from build123d import *

# Parameters (mm, degrees)
SKETCH1_W           = 15.24
SKETCH1_H           = 20.066
SKETCH1_W_2         = 5.588
SKETCH1_H_2         = 9.906
BOSS_EXTRUDE1_DEPTH = 3.175
CUT_EXTRUDE1_REACH  = 14.993
SKETCH2_R           = 1.3


with BuildPart() as part:
    # Sketch1 → Boss-Extrude1 (new body)
    with BuildSketch(Plane.XY):
        Rectangle(SKETCH1_W, SKETCH1_H)
        Rectangle(SKETCH1_W_2, SKETCH1_H_2, mode=Mode.SUBTRACT)
    extrude(amount=BOSS_EXTRUDE1_DEPTH)

    # Sketch2 → Cut-Extrude1 (cut, up to next)
    with BuildSketch(Plane.XY.offset(3.175), mode=Mode.PRIVATE) as cut_extrude1_sk1:
        with Locations((-5.207, 7.112)):
            Circle(SKETCH2_R)
    cut_extrude1_tool1 = extrude(cut_extrude1_sk1.sketch, amount=-CUT_EXTRUDE1_REACH, mode=Mode.PRIVATE) & part.part
    # Sketch2 → Cut-Extrude1 (cut, up to next)
    with BuildSketch(Plane.XY.offset(3.175), mode=Mode.PRIVATE) as cut_extrude1_sk2:
        with Locations((5.207, 7.112)):
            Circle(SKETCH2_R)
    cut_extrude1_tool2 = extrude(cut_extrude1_sk2.sketch, amount=-CUT_EXTRUDE1_REACH, mode=Mode.PRIVATE) & part.part
    # Sketch2 → Cut-Extrude1 (cut, up to next)
    with BuildSketch(Plane.XY.offset(3.175), mode=Mode.PRIVATE) as cut_extrude1_sk3:
        with Locations((5.207, -7.112)):
            Circle(SKETCH2_R)
    cut_extrude1_tool3 = extrude(cut_extrude1_sk3.sketch, amount=-CUT_EXTRUDE1_REACH, mode=Mode.PRIVATE) & part.part
    # Sketch2 → Cut-Extrude1 (cut, up to next)
    with BuildSketch(Plane.XY.offset(3.175), mode=Mode.PRIVATE) as cut_extrude1_sk4:
        with Locations((-5.207, -7.112)):
            Circle(SKETCH2_R)
    cut_extrude1_tool4 = extrude(cut_extrude1_sk4.sketch, amount=-CUT_EXTRUDE1_REACH, mode=Mode.PRIVATE) & part.part
    add(cut_extrude1_tool1.solids().sort_by_distance((-5.207, 7.112, 3.175))[0], mode=Mode.SUBTRACT)
    add(cut_extrude1_tool2.solids().sort_by_distance((5.207, 7.112, 3.175))[0], mode=Mode.SUBTRACT)
    add(cut_extrude1_tool3.solids().sort_by_distance((5.207, -7.112, 3.175))[0], mode=Mode.SUBTRACT)
    add(cut_extrude1_tool4.solids().sort_by_distance((-5.207, -7.112, 3.175))[0], mode=Mode.SUBTRACT)


solid = part.part
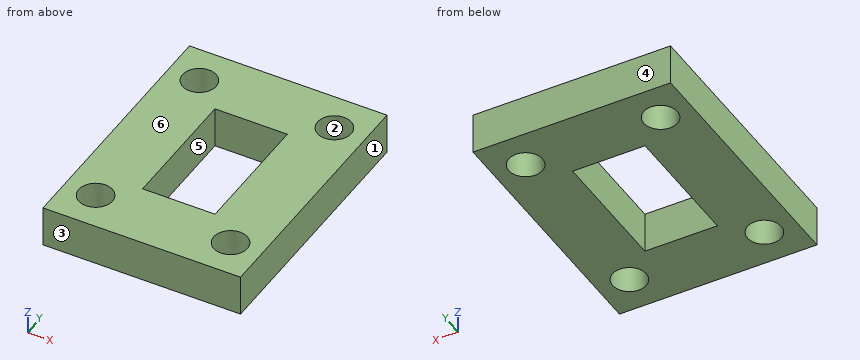
Part model, mm, in its own coordinate system. Face numbers are marked on the shaded views. A direction names the side the tool comes from. Coordinates: 2 decimals unless noted, no trailing zeros. Write each loop counter-clockwise with the first axis right and the second up, starting at its lowest first coordinate (ties: lowest second). Pieces come first, ordered by that corner, then holes. Notation, with made-up numbers: (-4, 12) - (27, 12) arc R5 cw to (27, 17) - close; hole circle Ø8 at (-10, -18.75). An arc over 180 degrees is marked (long way). Put each result on its own line as item: value.
1. 3-axis set-ups, long thin cutter, end or side, ignore diameter. For the marked faces 5 and 6: which of +Z, -Z, +X, -X, +Y, -Y reach the whole face in a straight line?
Final values:
face 5: +Z, -Z
face 6: +Z, +X, -X, +Y, -Y
2. Band-saw the part on D-D (x = 5). Write the cut outline in (y, z) (3 decimals).
Final values:
outline: (-10.033, 0) - (-8.395, 0) - (-8.395, 3.175) - (-10.033, 3.175) - close; (-5.829, 0) - (5.829, 0) - (5.829, 3.175) - (-5.829, 3.175) - close; (8.395, 0) - (10.033, 0) - (10.033, 3.175) - (8.395, 3.175) - close
3. Two-plate mould, pull along Y, no slides. Class the marked faces 1, 2, 3 and 4: +Y half, -Y half, draft (parallel to the pull), parting line (faces both ways), or undercut.
Final values:
face 1: draft
face 2: undercut
face 3: -Y half
face 4: +Y half
4. Band-saw the part on A-A (y = -1.5). Write the cut outline in (x, z) (3 decimals).
Final values:
outline: (-7.62, 0) - (-2.794, 0) - (-2.794, 3.175) - (-7.62, 3.175) - close; (2.794, 0) - (7.62, 0) - (7.62, 3.175) - (2.794, 3.175) - close
5. Band-saw the part on B-B (x = -1.5). Write the cut outline in (y, z) (3 decimals).
Final values:
outline: (-10.033, 0) - (-4.953, 0) - (-4.953, 3.175) - (-10.033, 3.175) - close; (4.953, 0) - (10.033, 0) - (10.033, 3.175) - (4.953, 3.175) - close
6. Flat gauge pin, fed straight in: pin 1 Ø2 at (x, y) = (5.207, 7.112) entering from +Z. Where does the tip first touch, or does it go through?
Final values:
pin 1: passes through
7. Band-saw the part on C-C (z = 2.6). Write the cut outline in (x, y), then the cut area to 3 significant figures.
Final values:
outline: (-7.62, -10.03) - (7.62, -10.03) - (7.62, 10.03) - (-7.62, 10.03) - close; hole circle Ø2.6 at (-5.21, -7.11); hole circle Ø2.6 at (-5.21, 7.11); hole (-2.79, -4.95) - (2.79, -4.95) - (2.79, 4.95) - (-2.79, 4.95) - close; hole circle Ø2.6 at (5.21, -7.11); hole circle Ø2.6 at (5.21, 7.11)
area: 229 mm²
8. Probe line 1 along Y through (x, z) = (5.25, 1.9); line 2 along X through (y, z) = (-7, 2.05); line 3 along X through (y, z) = (0, 0.9). List the from-to ranges inside material, lowest first. Write a range as [from, to].
Final values:
line 1: y = [-10.03, -8.41], [-5.81, 5.81], [8.41, 10.03]
line 2: x = [-7.62, -6.5], [-3.91, 3.91], [6.5, 7.62]
line 3: x = [-7.62, -2.79], [2.79, 7.62]
